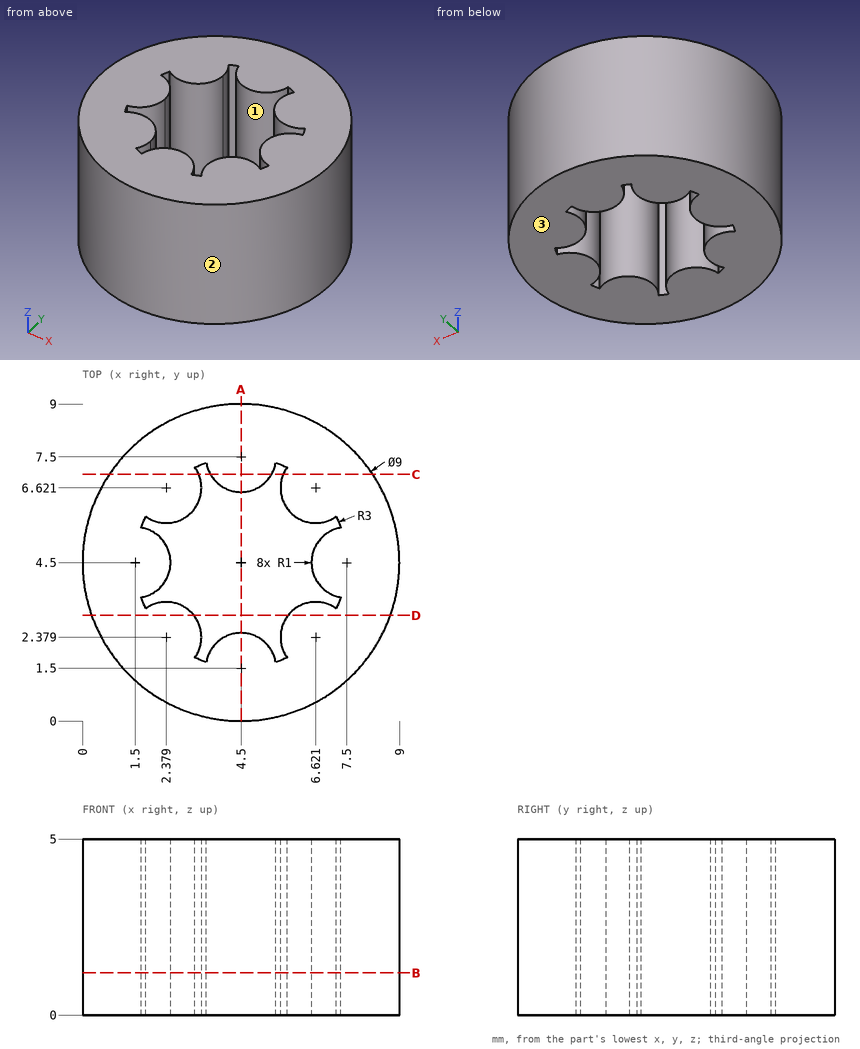
Geometry check sheet. Reference: drawing and pictorial views, mm from the part's lowest x, y, z. Coordinates: 2 decimals unless noted, no trailing zeros. Loops run counter-clockwise (first coordinate to the right, second up) from the corner with the lowest first, then second, coordinate; pieces in that order, holes last.
1) Sectioned sample at D-D (y = 3). Record the boundary of the cut face in (x, z).
2) Material ranges on probe 1 along X at (y, z) = (2.25, 3.75) (1 decimal); probe 2 along X at (y, z) = (1.75, 0.7) (1 decimal); probe 3 along Y at (x, z) = (2, 4.5) (1 decimal), recorded low to high.
3) Sectioned sample at A-A (x = 4.5). Record the boundary of the cut face in (y, z).
4) Gauge pin test, flat ends, axial feed: pin 1 (1.5 mm diameter, centred on y = 3.5, z = 1.5, fed in from -X); pin 2 (1 mm diameter, centred on x = 1, z = 2.5, fed in from -Y) (1 decimal); pin 3 (1.5 mm diameter, centred on x = 3.5, z = 1.5, fed in from -Y). Record the tip position at first contact, or that the pin passes through.
5) Sectioned sample at B-B (z = 1.2). Record the boundary of the cut face in (x, y).
6) Sectioned sample at C-C (y = 7). Record the boundary of the cut face in (x, z).
7) Release check for a two-part mould opening along Y. For the marked faces 1, 2 and 3 record: released by +Y, released by -Y, zero draft, split by the parting line, or undercut.
Check sheet entries:
1. outline: (0.26, 0) - (3.16, 0) - (3.16, 5) - (0.26, 5) - close; (5.84, 0) - (8.74, 0) - (8.74, 5) - (5.84, 5) - close
2. probe 1: x = 0.6 to 3.4, 3.8 to 5.2, 5.6 to 8.4
2. probe 2: x = 0.9 to 3.3, 3.5 to 5.5, 5.7 to 8.1
2. probe 3: y = 0.8 to 3.3, 3.6 to 5.4, 5.7 to 8.2
3. outline: (0, 0) - (2.5, 0) - (2.5, 5) - (0, 5) - close; (6.5, 0) - (9, 0) - (9, 5) - (6.5, 5) - close
4. pin 1: stops at x = 0.01
4. pin 2: stops at y = 1.1
4. pin 3: stops at y = 0.01
5. outline: circle Ø9 at (4.5, 4.5); hole (1.67, 3.51) arc R3 ccw to (1.8, 3.19) arc R1 cw to (3.19, 1.8) arc R3 ccw to (3.51, 1.67) arc R1 cw to (5.49, 1.67) arc R3 ccw to (5.81, 1.8) arc R1 cw to (7.2, 3.19) arc R3 ccw to (7.33, 3.51) arc R1 cw to (7.33, 5.49) arc R3 ccw to (7.2, 5.81) arc R1 cw to (5.81, 7.2) arc R3 ccw to (5.49, 7.33) arc R1 cw to (3.51, 7.33) arc R3 ccw to (3.19, 7.2) arc R1 cw to (1.8, 5.81) arc R3 ccw to (1.67, 5.49) arc R1 cw to start
6. outline: (0.76, 0) - (3.3, 0) - (3.3, 5) - (0.76, 5) - close; (3.63, 0) - (5.37, 0) - (5.37, 5) - (3.63, 5) - close; (5.7, 0) - (8.24, 0) - (8.24, 5) - (5.7, 5) - close
7. face 1: undercut
7. face 2: split by the parting line
7. face 3: zero draft
